The listing builds one solid part. Answer for the finished solid, in the listing's coordinates (mm). Face numbers are marked on the shaded views. A direction names the side the tool comes from. Give positions to 0.01 mm unless a question says otherwise; leave off trailing zeros. Write each loop counter-clockwise with the first axis right and the second up, starting at its lowest first coordinate (ties: lowest second). Pieces come first, ordered by that corner, then holes. Notation, with made-up numbers: (62, 50) - (91, 50) arc R19 cw to (91, 83) - close; hole circle Ø1 at (85.5, -18). An arc over 180 degrees is marked (long way). One line per question, with ' | ' between items. Start each with the question number.
1. Find the intervals of material crossed by L1, parallel to X at y = 7.5, z = 2.75; L2, parallel to Y at x = 6.5, z = 6.25; L3, parallel to X at y = 6.25, z = 6.75, in increasing order. Write a range as from..to.
2. The mould has two halves that part along Y. Classify the marked faces 1, 2, 3 and 4: +Y half, -Y half, draft (parallel to the pull), parting line (faces both ways), or undercut.
3. A cutting plane is placed at A-A (x = 6.75). Determine the outline of the cut face in (y, z), then the cut area to 3 significant figures.
4. A cutting plane is placed at B-B (y = 6.25). Determine the outline of the cut face in (x, z), then the cut area to 3 significant figures.
5. For the marked faces 5 and 6, determine the directions among +Z, -Z, +X, -X, +Y, -Y from which every point of the face is accessible in a straight line to the end or side of a thin tool.
6. Given P1, Ø3, axis at y = 5.5, z = -2, coming from the -X side; P2, Ø0.5, axis at x = 5.5, z = -1, coming from the +Y side; P3, Ø1, axis at x = 1.5, z = -1, coming from the +Y side; P4, Ø1.5, axis at x = 2.5, y = 14, coming from the -Z side, each flat-ended and moving along its own axis, determine where each tip first touches the part or whether it passes through.
7. A cutting plane is placed at C-C (z = -0.75). State how many separate pieces and enclosed holes the cut face has, then the cut area to 3 significant figures.
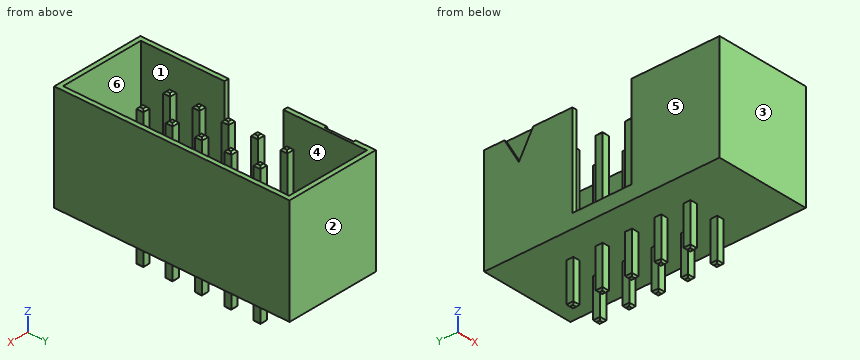
```python
from build123d import *

# Parameters (mm, degrees)
ESQUISSE1_W             = 8.2
ESQUISSE1_H             = 20.4
BOSS_EXTRU_1_DEPTH      = 9.2
ESQUISSE2_W             = 7.4
ESQUISSE2_H             = 19.6
ENL_V_MAT_EXTRU_1_DEPTH = 8
ESQUISSE3_W             = 0.6
ESQUISSE3_H             = 0.6
BOSS_EXTRU_2_DEPTH      = 3.5
BOSS_EXTRU_2_DEPTH_BACK = 8.5
CHANFREIN1_SIZE         = 0.15
ESQUISSE4_W             = 0.4
ESQUISSE4_H             = 5.1
ENL_V_MAT_EXTRU_2_DEPTH = 8
ENL_V_MAT_EXTRU_3_DEPTH = 0.2


with BuildPart() as part:
    # Esquisse1 → Boss.-Extru.1 (new body)
    with BuildSketch(Plane.XY):
        with Locations((4.1, 10.2)):
            Rectangle(ESQUISSE1_W, ESQUISSE1_H)
    extrude(amount=BOSS_EXTRU_1_DEPTH)

    # Esquisse2 → Enlèv. mat.-Extru.1 (cut)
    with BuildSketch(Plane.XY.offset(9.2)):
        with Locations((4.1, 10.2)):
            Rectangle(ESQUISSE2_W, ESQUISSE2_H)
    extrude(amount=-ENL_V_MAT_EXTRU_1_DEPTH, mode=Mode.SUBTRACT)

    # Esquisse3 → Boss.-Extru.2 (add, two sides)
    with BuildSketch(Plane(origin=(0, 0, 0), x_dir=(-1, 0, 0), z_dir=(0, 0, -1))) as boss_extru_2_sk:
        with Locations((-5.37, 15.28)):
            Rectangle(ESQUISSE3_W, ESQUISSE3_H)
        with Locations((-2.83, 15.28)):
            Rectangle(ESQUISSE3_W, ESQUISSE3_H)
        with Locations((-5.37, 12.74)):
            Rectangle(ESQUISSE3_W, ESQUISSE3_H)
        with Locations((-2.83, 12.74)):
            Rectangle(ESQUISSE3_W, ESQUISSE3_H)
        with Locations((-5.37, 10.2)):
            Rectangle(ESQUISSE3_W, ESQUISSE3_H)
        with Locations((-2.83, 10.2)):
            Rectangle(ESQUISSE3_W, ESQUISSE3_H)
        with Locations((-5.37, 7.66)):
            Rectangle(ESQUISSE3_W, ESQUISSE3_H)
        with Locations((-2.83, 7.66)):
            Rectangle(ESQUISSE3_W, ESQUISSE3_H)
        with Locations((-5.37, 5.12)):
            Rectangle(ESQUISSE3_W, ESQUISSE3_H)
        with Locations((-2.83, 5.12)):
            Rectangle(ESQUISSE3_W, ESQUISSE3_H)
    extrude(amount=BOSS_EXTRU_2_DEPTH)
    extrude(boss_extru_2_sk.sketch, amount=-BOSS_EXTRU_2_DEPTH_BACK)

    # Chanfrein1
    chanfrein1_edges = [part.edges().sort_by_distance(p)[0] for p in [
        (5.07, 10.2, 8.5),
        (5.37, 9.9, 8.5),
        (5.67, 10.2, 8.5),
        (5.37, 10.5, 8.5),
        (5.07, 10.2, -3.5),
        (5.37, 10.5, -3.5),
        (5.67, 10.2, -3.5),
        (5.37, 9.9, -3.5),
        (2.53, 10.2, 8.5),
        (2.83, 9.9, 8.5),
        (3.13, 10.2, 8.5),
        (2.83, 10.5, 8.5),
        (2.53, 10.2, -3.5),
        (2.83, 10.5, -3.5),
        (3.13, 10.2, -3.5),
        (2.83, 9.9, -3.5),
        (5.07, 7.66, 8.5),
        (5.37, 7.36, 8.5),
        (5.67, 7.66, 8.5),
        (5.37, 7.96, 8.5),
        (5.07, 7.66, -3.5),
        (5.37, 7.96, -3.5),
        (5.67, 7.66, -3.5),
        (5.37, 7.36, -3.5),
        (2.53, 7.66, 8.5),
        (2.83, 7.36, 8.5),
        (3.13, 7.66, 8.5),
        (2.83, 7.96, 8.5),
        (2.53, 7.66, -3.5),
        (2.83, 7.96, -3.5),
        (3.13, 7.66, -3.5),
        (2.83, 7.36, -3.5),
        (5.07, 5.12, 8.5),
        (5.37, 4.82, 8.5),
        (5.67, 5.12, 8.5),
        (5.37, 5.42, 8.5),
        (5.07, 5.12, -3.5),
        (5.37, 5.42, -3.5),
        (5.67, 5.12, -3.5),
        (5.37, 4.82, -3.5),
        (2.53, 5.12, 8.5),
        (2.83, 4.82, 8.5),
        (3.13, 5.12, 8.5),
        (2.83, 5.42, 8.5),
        (2.53, 5.12, -3.5),
        (2.83, 5.42, -3.5),
        (3.13, 5.12, -3.5),
        (2.83, 4.82, -3.5),
        (5.07, 15.28, 8.5),
        (5.37, 14.98, 8.5),
        (5.67, 15.28, 8.5),
        (5.37, 15.58, 8.5),
        (5.07, 15.28, -3.5),
        (5.37, 15.58, -3.5),
        (5.67, 15.28, -3.5),
        (5.37, 14.98, -3.5),
        (2.53, 15.28, 8.5),
        (2.83, 14.98, 8.5),
        (3.13, 15.28, 8.5),
        (2.83, 15.58, 8.5),
        (2.53, 15.28, -3.5),
        (2.83, 15.58, -3.5),
        (3.13, 15.28, -3.5),
        (2.83, 14.98, -3.5),
        (5.07, 12.74, 8.5),
        (5.37, 12.44, 8.5),
        (5.67, 12.74, 8.5),
        (5.37, 13.04, 8.5),
        (5.07, 12.74, -3.5),
        (5.37, 13.04, -3.5),
        (5.67, 12.74, -3.5),
        (5.37, 12.44, -3.5),
        (2.53, 12.74, 8.5),
        (2.83, 12.44, 8.5),
        (3.13, 12.74, 8.5),
        (2.83, 13.04, 8.5),
        (2.53, 12.74, -3.5),
        (2.83, 13.04, -3.5),
        (3.13, 12.74, -3.5),
        (2.83, 12.44, -3.5),
    ]]
    chamfer(chanfrein1_edges, length=CHANFREIN1_SIZE)

    # Esquisse4 → Enlèv. mat.-Extru.2 (cut)
    with BuildSketch(Plane.XY.offset(9.2)):
        with Locations((0.2, 10.2)):
            Rectangle(ESQUISSE4_W, ESQUISSE4_H)
    extrude(amount=-ENL_V_MAT_EXTRU_2_DEPTH, mode=Mode.SUBTRACT)

    # Esquisse5 → Enlèv. mat.-Extru.3 (cut)
    with BuildSketch(Plane.ZY):
        Polygon((9.2, 18.65), (9.2, 16.15), (7.034936491, 17.4), align=None)
    extrude(amount=-ENL_V_MAT_EXTRU_3_DEPTH, mode=Mode.SUBTRACT)


solid = part.part
```
Determined:
1) L1: 0..0.4, 2.53..3.13, 5.07..5.67, 7.8..8.2 | L2: 0..0.4, 20..20.4 | L3: 0..0.4, 7.8..8.2
2) face 1: undercut | face 2: +Y half | face 3: -Y half | face 4: undercut
3) outline: (0, 0) - (20.4, 0) - (20.4, 9.2) - (20, 9.2) - (20, 1.2) - (0.4, 1.2) - (0.4, 9.2) - (0, 9.2) - close | area: 30.9 mm2
4) outline: (0, 0) - (8.2, 0) - (8.2, 9.2) - (7.8, 9.2) - (7.8, 1.2) - (0.4, 1.2) - (0.4, 9.2) - (0, 9.2) - close | area: 16.2 mm2
5) face 5: +Z, -Z, -X, +Y, -Y | face 6: +Z
6) P1: x = 2.53 | P2: y = 15.58 | P3: through | P4: z = 0
7) separate pieces: 10 | enclosed holes: 0 | area: 3.60 mm2
